Input: part model. Units: mm. Frame: model coordinates. Face numbers are marked on the shaded views. A direction names the side the tool comes from. Round coordinates to 2 decimals unless told otherwise and drop trailing zeros. Order: outer loops, then holes, each group sorted by start corner. A loop starts at its lowest first (then second) coordinate and runs counter-clockwise, first axis right, second up. Notation, with made-up numbers: (74, -12.75) -> (118, -12.75) arc R24 cw to (118, 10.25) -> close; hole circle Ø2 at (-18.75, 73). An arc over 180 degrees is marked (long way). Answer as CSV lines item,"result". Start each with the question number.
1) Section query D-D, the plane x = 9.75. Output: boundary loops of the cut face in (y, z).
2) Section query A-A, the plane x = 25.5. Output: boundary loops of the cut face in (y, z).
3) Line query: L1, parallel to X at y = -73, z = 1.85; L2, parallel to Z at x = 13.5, y = 6.25; L3, parallel to Y at x = 17.5, z = 4.3. Output: solid intervals per line, ascending.
4) Mould query, pull axis Y, two halves, no side actions, for the marked faces 1, 2 and 3. Classes: +Y half, -Y half, draft (parallel to the pull), parting line (faces both ways), or undercut.
5) First-contact query: P1, Ø1, axis at y = -47, z = 2, coming from the +X side; P2, Ø2.5, axis at y = -0.5, z = 3, coming from the +X side; P3, Ø2.5, axis at y = -72, z = 2.5, coming from the +X side. Flat tips, straight axial feed; report the tip coordinate or a pass-through.
6) Section query C-C, the plane x = 15.75. Output: boundary loops of the cut face in (y, z), and give its area (4 significant figures).
7) Access query for the marked faces 4 and 5. Directions: +Z, -Z, +X, -X, +Y, -Y. A direction counts if a zero-diameter tool reaches every point of the face in a straight line with its end or side. Return the directions, or none.
8) Section query B-B, the plane y = -73. Output: boundary loops of the cut face in (x, z), and give its area (3 significant figures).
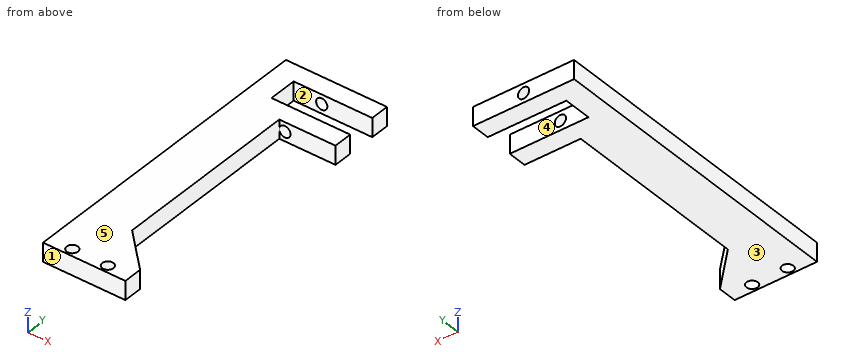
```python
from build123d import *

# Parameters (mm, degrees)
F0_R     = 1.5
F1_DEPTH = 5
F2_SIZE  = 9.99999
F4_DEPTH = 25


# Not quite as in the source:
# - a fillet or chamfer is up to 0.001 mm smaller than in the source, because OpenCascade refuses the exact size


with BuildPart() as f1:
    # F0 (on Top) → F1 (new body)
    with BuildSketch(Plane.XY):
        Polygon((0, 7.5), (0, 0), (0, -75), (11, -75), (22, -75), (22, -60), (12, -60), (12, -10), (27, -10), (27, -5), (6, -5), (6, 2.5), (27, 2.5), (27, 7.5), align=None)
        with Locations((6.25, -73)):
            Circle(F0_R, mode=Mode.SUBTRACT)
        with BuildLine():
            ThreePointArc((17.25, -73), (15.75, -74.5), (14.25, -73))
            ThreePointArc((14.25, -73), (15.75, -71.5), (17.25, -73))
        make_face(mode=Mode.SUBTRACT)
    extrude(amount=F1_DEPTH)

    # F2 (size 10 in the source; OpenCascade refuses exactly that, so slightly less here)
    f2_edges = [f1.edges().sort_by_distance(p)[0] for p in [
        (22, -60, 2.5),
    ]]
    chamfer(f2_edges, length=F2_SIZE)

    # F3 (on face) → F4 (cut)
    with BuildSketch(Plane(origin=(0, 7.5, 0), x_dir=(-1, 0, 0), z_dir=(0, 1, 0))):
        with BuildLine():
            ThreePointArc((-15, 2.5), (-13.5, 1), (-12, 2.5))
            Line((-12, 2.5), (-15, 2.5))
        make_face()
        with BuildLine():
            Line((-15, 2.5), (-12, 2.5))
            ThreePointArc((-12, 2.5), (-13.5, 4), (-15, 2.5))
        make_face()
    extrude(amount=-F4_DEPTH, mode=Mode.SUBTRACT)


solid = f1.part
```
Findings:
1,outline,"(-75, 0) -> (-5, 0) -> (-5, 5) -> (-75, 5) -> close; (2.5, 0) -> (7.5, 0) -> (7.5, 5) -> (2.5, 5) -> close"
2,outline,"(-10, 0) -> (-5, 0) -> (-5, 5) -> (-10, 5) -> close; (2.5, 0) -> (7.5, 0) -> (7.5, 5) -> (2.5, 5) -> close"
3,L1,"x = 0 to 4.75, 7.75 to 14.25, 17.25 to 22"
3,L2,"z = 0 to 1, 4 to 5"
3,L3,"y = -75 to -65.5, -10 to -5, 2.5 to 7.5"
4,face 1,"-Y half"
4,face 2,"undercut"
4,face 3,"draft"
5,P1,"stops at x = 12"
5,P2,"stops at x = 6"
5,P3,"stops at x = 22"
6,outline,"(-75, 0) -> (-74.5, 0) -> (-74.5, 5) -> (-75, 5) -> close; (-71.5, 0) -> (-63.75, 0) -> (-63.75, 5) -> (-71.5, 5) -> close; (-10, 0) -> (-5, 0) -> (-5, 5) -> (-10, 5) -> close; (2.5, 0) -> (7.5, 0) -> (7.5, 5) -> (2.5, 5) -> close"
6,area,"91.25 mm^2"
7,face 4,"+Z, -Z, +X"
7,face 5,"+Z, +X, -X, +Y, -Y"
8,outline,"(0, 0) -> (4.75, 0) -> (4.75, 5) -> (0, 5) -> close; (7.75, 0) -> (14.25, 0) -> (14.25, 5) -> (7.75, 5) -> close; (17.25, 0) -> (22, 0) -> (22, 5) -> (17.25, 5) -> close"
8,area,"80.0 mm^2"
